Read the model definition and answer for the solid it produces. Units are mm, in the model's axes. Face numbers are marked on the shaded views. A direction names the side the tool comes from. Round coordinates to 2 decimals unless told otherwise and drop trailing zeros. Write each loop counter-clockwise with the first axis right and the second up, starting at its lowest first coordinate (ties: lowest second). Pieces come first, ordered by that corner, then holes. Notation, with made-up numbers: (80.5, -34.75) - (104.5, -34.75) arc R15 cw to (104.5, -28.75) - close; hole circle Ø9 at (-18, -13). An arc over 180 degrees is marked (long way). One line per item, written item: value. Start each with the question number.
(1) Flat-ended cylindrical pins translate along their axes: pin 1 Ø1.5 at (x, y) = (0.5, -4.5) entering from -Z; pin 2 Ø6 at (y, z) = (-6, 4) entering from -X; pin 3 Ø1.5 at (x, y) = (7, -3) entering from -Z. Find the tip coordinate at first contact, or state that the pin passes through.
(2) A cutting plane is placed at A-A, the plane z = 0. Determine the outline of the cut face in (x, y), plus the area to 4 significant figures.
(3) Find the intervals of material crossed by L1, parallel to X at y = -2.75, z = -6; L2, parallel to X at y = -3, z = 7; L3, parallel to Z at x = 3.75, y = 5 (3 decimals), in increasing order.
(4) A cutting plane is placed at C-C, the plane x = 8.75. Determine the outline of the cut face in (y, z).
(5) For the marked faces 1 and 2, determine the directions among +Z, -Z, +X, -X, +Y, -Y from which every point of the face is accessible in a straight line to the end or side of a thin tool.
(6) A cutting plane is placed at D-D, the plane x = -2. Determine the outline of the cut face in (y, z).
from build123d import *


with BuildPart() as part:
    # Sketch_Tip_Profile → Tip_Revolve_D16x10_Stud_M6x12 (revolve)
    with BuildSketch(Plane.XY, mode=Mode.PRIVATE) as tip_revolve_d16x10_stud_m6x12_sk:
        Polygon((-12, 0), (-12, 2.5), (-11.5, 3), (0, 3), (0, 8), (9.5, 8), (10, 7.5), (10, 0), align=None)
    revolve(tip_revolve_d16x10_stud_m6x12_sk.sketch.rotate(Axis((-15, 0, 0), (1, 0, 0)), 90), axis=Axis((-15, 0, 0), (1, 0, 0)))


solid = part.part
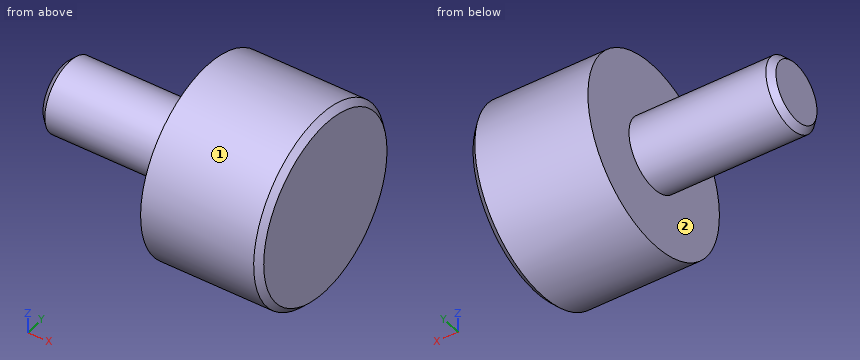
Here are the results:
1. pin 1: z = -7.07
1. pin 2: x = 0
1. pin 3: z = -7.68
2. outline: (-12, -2.5) - (-11.5, -3) - (0, -3) - (0, -8) - (9.5, -8) - (10, -7.5) - (10, 7.5) - (9.5, 8) - (0, 8) - (0, 3) - (-11.5, 3) - (-12, 2.5) - close
2. area: 231.5 mm²
3. L1: 0 to 10
3. L2: 0 to 9.88
3. L3: -6.245 to 6.245
4. outline: circle Ø16 at (0, 0)
5. face 1: +X, -X
5. face 2: -X
6. outline: circle Ø6 at (0, 0)
